Autodesk Inventor part; units mm, degrees
ref_plane "YZ Plane" through (0, 0, 0) normal (1, 0, 0) x (0, 1, 0)
ref_plane "XZ Plane" through (0, 0, 0) normal (0, 1, 0) x (-1, 0, 0)
ref_plane "XY Plane" through (0, 0, 0) normal (0, 0, 1) x (1, 0, 0)
sketch "Sketch1" plane through (0, 0, 0) normal (0, 0, 1) x (1, 0, 0)
  circle A0 centre (0, 0) radius 12.7
  circle A1 centre (0, 0) radius 4
  circle A2 centre (9.525, 0) radius 1.5
  circle A3 centre (-4.7625, 8.2489) radius 1.5
  circle A4 centre (-4.7625, -8.2489) radius 1.5
  dimension "d0" = 25.4
  dimension "d1" = 8
  dimension "d2" = 3
  dimension "d6" = 360
  dimension "d25" = 9.525
extrude "Extrusion1" add sketch "Sketch1" along normal blind 12.7
sketch "Sketch2" plane through (0, 0, 12.7) normal (0, 0, 1) x (1, 0, 0)
  line L0 (-12.7, 0.5) -> (-3.9686, 0.5)
  line L1 (-3.9686, 0.5) -> (-3.9686, -0.5)
  line L2 (-3.9686, -0.5) -> (-12.7, -0.5)
  line L3 (-12.7, -0.5) -> (-12.7, 0.5)
  circle A0 centre (0, 0) radius 12.7 construction
  circle A1 centre (0, 0) radius 4 construction
  point P0 (-3.9686, 0)
  point P1 (-12.7, 0)
  dimension "d10" = 1
extrude "Extrusion2" cut sketch "Sketch2" against normal through all
sketch "Sketch3" plane through (-12.6902, 0.5, 12.7) normal (0, -1, 0) x (1, 0, 0)
  circle A0 centre (3, -3) radius 2
  circle A1 centre (3, -9.45) radius 2
  line L0 (25.3902, 0) -> (0, 0)
  line L1 (0, -12.7) -> (25.3902, -12.7)
  point P0 (12.6902, -12.7)
  point P1 (12.6902, -12.7)
  point P2 (12.6902, -12.7)
  point P3 (12.6902, -12.7)
  point P4 (12.6902, -12.7)
  dimension "d13" = 4
  dimension "d14" = 4
  dimension "d15" = 3
  dimension "d16" = 3
  dimension "d17" = 3.25
extrude "Extrusion3" cut sketch "Sketch3" along normal through all both and the other way through all
sketch "Sketch4" plane through (0, 0, 12.7) normal (0, 0, 1) x (1, 0, 0)
  circle A0 centre (0, 0) radius 7
  arc A1 (-12.6902, -0.5) -> (-12.6902, 0.5) centre (0, 0) ccw
  circle A2 centre (0, 0) radius 12.7
  dimension "d24" = 14
extrude "Extrusion4" cut sketch "Sketch4" against normal blind 6.2
sketch "Sketch5" plane through (0, 0, 0) normal (0, 1, 0) x (-1, 0, 0)
  circle A0 centre (0, 9.6) radius 1.5
  circle A1 centre (0, 3.25) radius 1.5
  line L0 (-12.7, 0) -> (-12.7, 6.5)
  line L1 (-7, 12.7) -> (-7, 6.5)
  point P0 (0, 0)
  point P1 (-12.7, 3.25)
  point P2 (-7, 9.6)
  dimension "d28" = 3
  dimension "d29" = 3
extrude "Extrusion5" cut sketch "Sketch5" against normal through all contours A0
thread "Thread2"
thread "Thread3"
properties part number "AA056" material "Aluminum 6061"
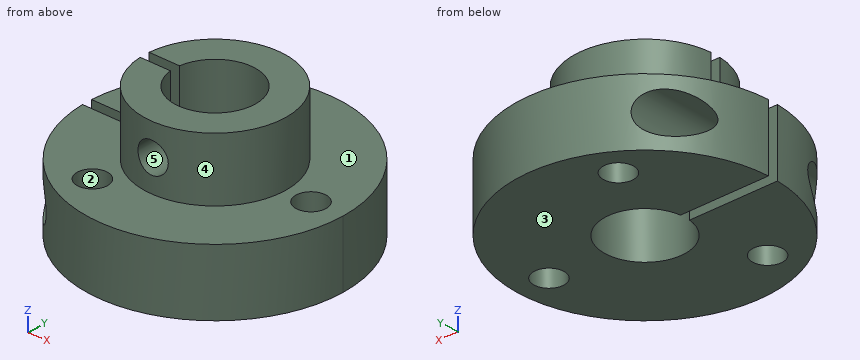
CAD build for the part. Positions are in the model's coordinates, mm. Face numbers are marked on the shaded views. A direction names the side the tool comes from. Round coordinates to 2 decimals unless told otherwise and drop trailing zeros. Order: outer loops, then holes, each group sorted by start corner. A loop starts at its lowest first (then second) coordinate and runs counter-clockwise, first axis right, second up. Notation, with made-up numbers: (36.5, 49.5) - (83.5, 49.5) arc R16 ccw to (83.5, 80.5) - close; hole circle Ø5 at (40.25, 84.5). An arc over 180 degrees is marked (long way). Answer as CSV lines item,"result". Start each with the question number.
1. Pull direction X, two halves, no side cores. Call the marked faces 3, 4 and 5: +X half, -X half, draft (parallel to the pull), parting line (faces both ways), or undercut.
2. Pin check, flat tips, straight feed: pin 1 (6.5 mm diameter, centred on x = -9.69, z = 3.25, fed in from +Y); pin 2 (2.5 mm diameter, centred on x = 0, z = 9.6, fed in from +Y); pin 3 (4.5 mm diameter, centred on x = -6.5, z = 4.5, fed in from +Y); pin 4 (3.5 mm diameter, centred on x = -9.69, z = 3.25, fed in from +Y). Stop position of each tip, or through.
3. Saw through at D-D, the plane y = -7.5. Write the cut outline in (x, z), and give its area (3 significant figures).
4. Drill centre lines: L1, parallel to Y at x = 0, z = 5.25; L2, parallel to Z at x = 0, y = -5.2; L3, parallel to X at y = 1, z = 1.75. Where is each one in solid material? Low to high. Write a range as [from, to].
5. Tool access for the marked faces 1 and 2: list every direction of +Z, -Z, +X, -X, +Y, -Y with a clear straight run to the whole face (end or side of a thin tool).
6. Saw through at C-C, the plane z = 4. Write the cut outline in (x, y) (1 decimal).
7. Saw through at B-B, the plane y = 2.75. Write the cut outline in (x, z), and give its area (3 significant figures).
8. Saw through at A-A, the plane x = 0. Write the cut outline in (y, z).
Model answer:
1,face 3,"draft"
1,face 4,"parting line"
1,face 5,"undercut"
2,pin 1,"stops at y = 10.95"
2,pin 2,"stops at y = 7"
2,pin 3,"stops at y = 11.97"
2,pin 4,"passes through"
3,outline,"(-10.25, 0) - (-6.06, 0) - (-6.06, 6.5) - (-10.25, 6.5) - (-10.25, 5.17) arc R2 cw (long way) to (-10.25, 1.33) - close; (-3.46, 0) - (10.25, 0) - (10.25, 6.5) - (-3.46, 6.5) - close"
3,area,"108 mm²"
4,L1,"y = [-12.7, -4], [4, 12.7]"
4,L2,"z = [0, 8.1], [11.1, 12.7]"
4,L3,"x = [-12.66, -11.01], [-8.37, -3.87], [3.87, 8.41], [10.64, 12.66]"
5,face 1,"+Z"
5,face 2,"+Z, -Z"
6,outline,"(-12.7, -0.5) arc R12.7 ccw to (-11.5, -5.3) - (-11.5, -0.5) - close; (-12.7, 0.5) - (-11.5, 0.5) - (-11.5, 5.3) arc R12.7 ccw to start; (-7.8, -10) arc R12.7 ccw (long way) to (-7.8, 10) - (-7.8, 0.5) - (-4, 0.5) arc R4 cw (long way) to (-4, -0.5) - (-7.8, -0.5) - close; hole circle Ø3 at (-4.8, -8.2); hole circle Ø3 at (-4.8, 8.2); hole circle Ø3 at (9.5, 0)"
7,outline,"(-12.4, 0) - (-2.9, 0) - (-2.9, 12.7) - (-6.44, 12.7) - (-6.44, 6.5) - (-12.4, 6.5) - close; (2.9, 0) - (12.4, 0) - (12.4, 6.5) - (6.44, 6.5) - (6.44, 12.7) - (2.9, 12.7) - close; hole circle Ø4 at (-9.69, 3.25)"
7,area,"155 mm²"
8,outline,"(-12.7, 0) - (-4, 0) - (-4, 8.1) - (-7, 8.1) - (-7, 6.5) - (-12.7, 6.5) - close; (-7, 11.1) - (-4, 11.1) - (-4, 12.7) - (-7, 12.7) - close; (4, 0) - (12.7, 0) - (12.7, 6.5) - (7, 6.5) - (7, 12.7) - (4, 12.7) - close"
